Autodesk Inventor part; units mm, degrees
ref_plane "YZ Plane" through (0, 0, 0) normal (1, 0, 0) x (0, 1, 0)
ref_plane "XZ Plane" through (0, 0, 0) normal (0, 1, 0) x (-1, 0, 0)
ref_plane "XY Plane" through (0, 0, 0) normal (0, 0, 1) x (1, 0, 0)
sketch "Szkic1" plane through (0, 0, 0) normal (1, 0, 0) x (0, 1, 0)
  line L0 (-16, 16) -> (16, 16)
  line L1 (16, 16) -> (16, -16)
  line L2 (16, -16) -> (-16, -16)
  line L3 (-16, -16) -> (-16, 16)
  line L4 (-16, 16) -> (16, -16) construction
  line L5 (16, 16) -> (-16, -16) construction
  line L6 (0, 0) -> (12.7279, 12.7279) construction
  circle A0 centre (12.7279, 12.7279) radius 1.5
  line L7 (0, 0) -> (0, 7.3193) construction
  line L8 (0, 0) -> (3.8373, 0) construction
  circle A1 centre (-12.7279, 12.7279) radius 1.5
  circle A2 centre (12.7279, -12.7279) radius 1.5
  circle A3 centre (-12.7279, -12.7279) radius 1.5
  circle A4 centre (0, 0) radius 14
  dimension "d0" = 32
  dimension "d1" = 32
  dimension "d2" = 18
  dimension "d3" = 3
  dimension "d4" = 28
extrude "Wyciągnięcie proste1" add sketch "Szkic1" along normal blind 10
fillet "Zaokrąglenie1" radius 4 4 edges at (5, 16, 16) (5, 16, -16) (5, -16, 16) (5, -16, -16)
sketch "Szkic2" plane through (10, 0, 0) normal (1, 0, 0) x (0, 0, -1)
  circle A0 centre (0, 0) radius 3.5
  line L0 (0, 3.5) -> (-1, 3.5) construction
  line L1 (-1, 3.5) -> (1, 3.5) construction
  circle A1 centre (0, 0) radius 14 construction
  line L2 (0, 0) -> (0, 1.6463) construction
  arc A2 (-1, 3.3541) -> (-1.5597, 13.9129) centre (-31.1594, 7.0497) ccw
  arc A3 (1.5597, 13.9129) -> (1, 3.3541) centre (31.1594, 7.0497) ccw
  arc A4 (1.5597, 13.9129) -> (-1.5597, 13.9129) centre (0, 0) ccw
  dimension "d8" = 7
  dimension "d9" = 1
  dimension "d10" = 2
extrude "Wyciągnięcie proste2" add sketch "Szkic2" against normal blind 1 contours A0
sketch "Szkic3" plane through (10, 0, 0) normal (1, 0, 0) x (0, 0, -1)
  arc A0 (0.3871, 3.4785) -> (-0.53, 3.4596) centre (0, 0) ccw
  arc A1 (-9.0021, 10.722) -> (-9.443, 10.3358) centre (0, 0) ccw
  circle A2 centre (0, 0) radius 3.5
  line L0 (-0.53, 3.4596) -> (-9.443, 10.3358)
  circle A3 centre (0, 0) radius 14
  line L1 (0.3871, 3.4785) -> (-9.0021, 10.722)
extrude "Wyciągnięcie proste3" add sketch "Szkic3" against normal blind 1 contours A0 L0 A1 L1
pattern_circular "Szyk kołowy1" count 4 over 360 about axis through (10, 0, 0) along (-1, 0, 0) of "Wyciągnięcie proste3"
fillet "Zaokrąglenie2" radius 1 4 edges at (9.5, 3.4596, 0.53) (9.5, 0.53, -3.4596) (9.5, -0.53, 3.4596) (9.5, -3.4596, -0.53)
fillet "Zaokrąglenie3" radius 0.5 16 edges at (10, -14.8284, 14.8284) (10, -16, 0) (10, -14.8284, -14.8284) (10, 0, -16) (10, 14.8284, -14.8284) (10, 16, 0) (10, 14.8284, 14.8284) (10, 0, 16) (0, 14.8284, 14.8284) (0, 16, 0) (0, 14.8284, -14.8284) (0, 0, -16) (0, -14.8284, -14.8284) (0, -16, 0) (0, -14.8284, 14.8284) (0, 0, 16)
fillet "Zaokrąglenie4" radius 0.5 5 edges at (10, -13.9695, 0.9239) (10, -0.9239, -13.9695) (10, 13.155, 4.7902) (10, 12.8102, -5.6479) (10, 0.9239, 13.9695)
sketch "Szkic4" plane through (10, 0, 0) normal (1, 0, 0) x (0, 0, -1)
  circle A0 centre (-12.7279, 12.7279) radius 1.5
  circle A1 centre (-12.7279, 12.7279) radius 2
  circle A2 centre (12.7279, 12.7279) radius 1.5
  circle A3 centre (12.7279, 12.7279) radius 2
  circle A4 centre (12.7279, -12.7279) radius 1.5
  circle A5 centre (12.7279, -12.7279) radius 2
  circle A6 centre (-12.7279, -12.7279) radius 1.5
  circle A7 centre (-12.7279, -12.7279) radius 2
  point P0 (0, 0)
  dimension "d21" = 4
  dimension "d22" = 4
  dimension "d23" = 4
  dimension "d24" = 4
extrude "Wyciągnięcie proste4" cut sketch "Szkic4" against normal blind 1
properties part number "WIATRAK"
Read the model definition and answer for the solid it produces. Units are mm, in the model's axes. A direction names the side the tool comes from. Coordinates: 2 decimals unless noted, no trailing zeros. Loops run counter-clockwise (first coordinate to the right, second up) from the corner with the lowest first, then second, coordinate; pieces in that order, holes last. Notation, with made-up numbers: (57, -26.75) -> (67, -26.75) arc R31 cw to (67, 5.25) -> close; hole circle Ø9 at (5, 77). An arc over 180 degrees is marked (long way). Return JSON: item names as keys, results as strings.
Item 1: Find the intervals of material crossed by probe 1 along Y at (x, z) = (9.5, 11); probe 2 along Y at (x, z) = (3.75, 0); probe 3 along X at (y, z) = (-3.5, 0), in increasing order.
Answers:
{"probe 1": "y = -16 to -13.74, -11.72 to -8.66, 8.66 to 11.72, 13.74 to 16", "probe 2": "y = -16 to -14, 14 to 16", "probe 3": "x = 9 to 10"}
Item 2: Flat-ended cylindrical pins translate along their axes: P1, Ø3, axis at y = 12.5, z = 12.5, coming from the +X side; P2, Ø4, axis at y = -12.73, z = 12.73, coming from the -X side; P3, Ø17, axis at y = 4.5, z = 2.5, coming from the -X side. Find the tip coordinate at first contact, or state that the pin passes through.
Answers:
{"P1": "stops at x = 9", "P2": "stops at x = 0", "P3": "stops at x = 9"}
Item 3: Find section C-C (x = 8.25). Determine the outline of the cut face in (y, z), plus the area to 3 significant figures.
Answers:
{"outline": "(-16, -12) arc R4 ccw to (-12, -16) -> (12, -16) arc R4 ccw to (16, -12) -> (16, 12) arc R4 ccw to (12, 16) -> (-12, 16) arc R4 ccw to (-16, 12) -> close; hole circle Ø3 at (-12.73, -12.73); hole circle Ø3 at (-12.73, 12.73); hole circle Ø28 at (0, 0); hole circle Ø3 at (12.73, -12.73); hole circle Ø3 at (12.73, 12.73)", "area": "366 mm2"}
Item 4: For faces 5 (the cylindrical face through (9.493, -1.518, 3.711)), 6 (the flat face through (9, 0, 0)), 7 (the cylindrical face through (9.507, -11.376, 14.202)), determine the directions among +Z, -Z, +X, -X, +Y, -Y from which every point of the face is accessible in a straight line to the end or side of a thin tool.
Answers:
{"face 5": "+X, -X", "face 6": "-X", "face 7": "+X"}
Item 5: For a pull along Y with two mould halves and no side action, classify faces 1 (the flat face through (5, -16, 0)), 2 (the flat face through (0, -4, -14)), 3 (the flat face through (5, 16, 0)), 4 (the cylindrical face through (4.44, 11.23, 12.66)) as +Y half, -Y half, draft (parallel to the pull), parting line (faces both ways), or undercut.
Answers:
{"face 1": "-Y half", "face 2": "draft", "face 3": "+Y half", "face 4": "undercut"}
Item 6: Find section A-A (y = 0). Determine the outline of the cut face in (x, z), plus the area to 3 significant figures.
Answers:
{"outline": "(0, -15.5) arc R0.5 ccw to (0.5, -16) -> (9.5, -16) arc R0.5 ccw to (10, -15.5) -> (10, -14.5) arc R0.5 ccw to (9.5, -14) -> (0, -14) -> close; (0, 14) -> (9.5, 14) arc R0.5 ccw to (10, 14.5) -> (10, 15.5) arc R0.5 ccw to (9.5, 16) -> (0.5, 16) arc R0.5 ccw to (0, 15.5) -> close; (9, -3.78) -> (10, -3.78) -> (10, 3.78) -> (9, 3.78) -> close", "area": "47.2 mm2"}
Item 7: Find section D-D (z = 4). Count the separate pieces of the cut face and the enclosed holes in it, plus the area to 3 significant figures.
Answers:
{"separate pieces": "4", "enclosed holes": "0", "area": "53.3 mm2"}
